Can you work these out from the model? Positions are in its coordinate system, mm. Face numbers are marked on the shaded views. A direction names the side the tool comes from. Round coordinates to 2 decimals unless told otherwise and drop trailing zeros. Order: outer loops, then holes, each group sorted by start corner. A loop starts at its lowest first (then second) coordinate and runs counter-clockwise, first axis right, second up. Notation, with made-up numbers: (77.25, -32.5) - (88.25, -32.5) arc R18 ccw to (88.25, -19.5) - close; hole circle Ø1 at (-9.5, -1.75). An arc over 180 degrees is marked (long way). Write item = value, one per line.
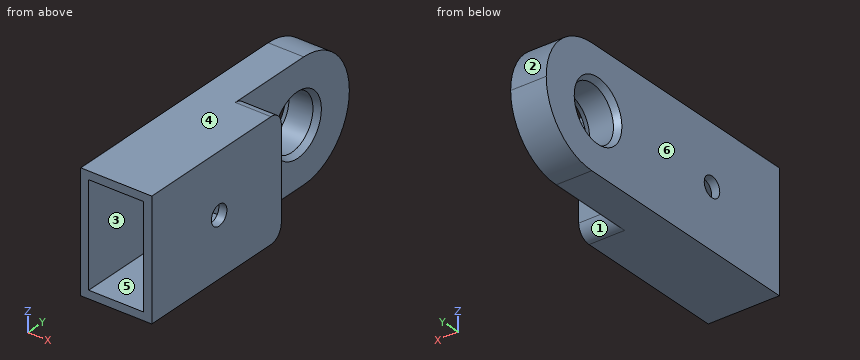
from build123d import *
from OCP.BRepFilletAPI import BRepFilletAPI_MakeChamfer

# Parameters (mm, degrees)
SKETCH1_W           = 10.6
SKETCH1_H           = 17.6
BOSS_EXTRUDE1_DEPTH = 25
SKETCH2_W           = 8.2
SKETCH2_H           = 15.2
CUT_EXTRUDE1_DEPTH  = 23
SKETCH4_W           = 5.3
SKETCH4_H           = 17.6
BOSS_EXTRUDE2_DEPTH = 20
CUT_EXTRUDE2_REACH  = 48.158
SKETCH5_R           = 4.1
FILLET1_R           = 8.8
FILLET2_R           = 2
SKETCH6_R           = 1.5
CUT_EXTRUDE3_DEPTH  = 48.061661679
CHAMFER1_SIZE       = 0.5
CHAMFER1_SIZE2      = 0.866025404


with BuildPart() as part:
    # Sketch1 → Boss-Extrude1 (new body)
    with BuildSketch(Plane(origin=(0, 0, 0), x_dir=(1, 0, 0), z_dir=(0, 1, 0))):
        Rectangle(SKETCH1_W, SKETCH1_H)
    extrude(amount=BOSS_EXTRUDE1_DEPTH)

    # Sketch2 → Cut-Extrude1 (cut)
    with BuildSketch(Plane.XZ):
        Rectangle(SKETCH2_W, SKETCH2_H)
    extrude(amount=-CUT_EXTRUDE1_DEPTH, mode=Mode.SUBTRACT)

    # Sketch4 → Boss-Extrude2 (add)
    with BuildSketch(Plane(origin=(0, 25, 0), x_dir=(1, 0, 0), z_dir=(0, 1, 0))):
        with Locations((-2.65, 0)):
            Rectangle(SKETCH4_W, SKETCH4_H)
    extrude(amount=BOSS_EXTRUDE2_DEPTH)

    # Sketch5 → Cut-Extrude2 (cut, up to next)
    with BuildSketch(Plane(origin=(0, 0, 0), x_dir=(0, 0, -1), z_dir=(1, 0, 0)), mode=Mode.PRIVATE) as cut_extrude2_sk1:
        with Locations((0, 35)):
            Circle(SKETCH5_R)
    cut_extrude2_tool1 = extrude(cut_extrude2_sk1.sketch, amount=-CUT_EXTRUDE2_REACH, mode=Mode.PRIVATE) & part.part
    add(cut_extrude2_tool1.solids().sort_by_distance((0, 35, 0))[0], mode=Mode.SUBTRACT)

    # Fillet1
    fillet1_edges = [part.edges().sort_by_distance(p)[0] for p in [
        (-2.65, 45, -8.8),
        (-2.65, 45, 8.8),
    ]]
    fillet(fillet1_edges, radius=FILLET1_R - 0.0001)  # a hair under: the kernel refuses the full size

    # Fillet2
    fillet2_edges = [part.edges().sort_by_distance(p)[0] for p in [
        (2.65, 25, 8.8),
        (2.65, 25, -8.8),
    ]]
    fillet(fillet2_edges, radius=FILLET2_R)

    # Sketch6 → Cut-Extrude3 (cut, through all)
    with BuildSketch(Plane(origin=(5.3, 0, 0), x_dir=(0, 0, -1), z_dir=(1, 0, 0))):
        with Locations((0, 13)):
            Circle(SKETCH6_R)
    extrude(amount=-CUT_EXTRUDE3_DEPTH, mode=Mode.SUBTRACT)

    # Chamfer1: one chamfer whose edges measure the first distance from different faces: ONE call of the kernel's chamfer builder (chamfer() names one face for all edges)
    chamfer1_edges_1 = [part.edges().sort_by_distance(p)[0] for p in [
        (0, 35, 4.1),
    ]]
    chamfer1_side_1 = [part.faces().sort_by_distance(p)[0] for p in [
        (0, 25.281737466, 0),
    ]]
    chamfer1_edges_2 = [part.edges().sort_by_distance(p)[0] for p in [
        (-5.3, 35, 4.1),
    ]]
    chamfer1_side_2 = [part.faces().sort_by_distance(p)[0] for p in [
        (-5.3, 20.674988238, 0),
    ]]
    chamfer1 = BRepFilletAPI_MakeChamfer(part.part.solid().wrapped)
    for e in chamfer1_edges_1:
        chamfer1.Add(CHAMFER1_SIZE, CHAMFER1_SIZE2, e.wrapped, chamfer1_side_1[0].wrapped)  # the first distance lies on this face
    for e in chamfer1_edges_2:
        chamfer1.Add(CHAMFER1_SIZE, CHAMFER1_SIZE2, e.wrapped, chamfer1_side_2[0].wrapped)  # the first distance lies on this face
    add(Compound.cast(chamfer1.Shape()), mode=Mode.REPLACE)


solid = part.part
(1) If we section it at A-A (y = 13): Write out the boundary of the cut face in (x, z), plus the area to 3 significant figures.
Computed:
outline = (-5.3, -8.8) - (5.3, -8.8) - (5.3, -1.5) - (4.1, -1.5) - (4.1, -7.6) - (-4.1, -7.6) - (-4.1, -1.5) - (-5.3, -1.5) - close; (-5.3, 1.5) - (-4.1, 1.5) - (-4.1, 7.6) - (4.1, 7.6) - (4.1, 1.5) - (5.3, 1.5) - (5.3, 8.8) - (-5.3, 8.8) - close
area = 54.7 mm^2
(2) Thinking about a two-plate mould opening in X: for the marked faces 3, 4, 5 and 6, which applies, +X half, -X half, draft (parallel to the pull), parting line (faces both ways), or undercut?
Computed:
face_3 = undercut
face_4 = draft
face_5 = undercut
face_6 = -X half
(3) If I drill on line 1 (X direction, y = 16, z = 3.75); line 2 (Z direction, x = -0.5, y = 13); line 3 (Y direction, x = 3, z = 4), over which ranges is the centre line in solid material (lowest first)? Write a range as from..to.
Computed:
line_1 = -5.3..-4.1, 4.1..5.3
line_2 = -8.8..-7.6, 7.6..8.8
line_3 = 23..25
(4) If we section it at D-D (z = 5.75): Write out the boundary of the cut face in (x, y), plus the area to 3 significant figures.
Computed:
outline = (-5.3, 0) - (-4.1, 0) - (-4.1, 23) - (4.1, 23) - (4.1, 0) - (5.3, 0) - (5.3, 25) - (0, 25) - (0, 42.86) - (-5.3, 42.86) - close
area = 171 mm^2
(5) Will these pins go through, and if not, where does the flat tip stop? P1, Ø5, axis at x = -1, z = -3, coming from the +Y side; P2, Ø5.5, axis at y = 37.5, z = 4, coming from the +X side; P3, Ø2.5, axis at y = 13, z = 0, coming from the -X side.
Computed:
P1 = 44.99
P2 = 0
P3 = through
(6) On a 3-axis mill with a long thin cutter (end or side, diameter ignored), from which of +Z, -Z, +X, -X, +Y, -Y can I reach the whole of each face in a straight line? I mean the marked faces 1 and 2. Say none if no direction works.
Computed:
face_1 = -Z, +X, +Y
face_2 = +Z, +X, -X, +Y
(7) If we section it at B-B (x = 3): Write out the boundary of the cut face in (y, z), plus the area to 3 significant figures.
Computed:
outline = (0, -8.8) - (23, -8.8) arc R2 ccw to (25, -6.8) - (25, 6.8) arc R2 ccw to (23, 8.8) - (0, 8.8) - (0, 7.6) - (23, 7.6) - (23, -7.6) - (0, -7.6) - close
area = 88.7 mm^2
(8) If we section it at C-C (y = 35): Write out the boundary of the cut face in (x, z).
Computed:
outline = (-5.3, -8.8) - (0, -8.8) - (0, -4.6) - (-0.87, -4.1) - (-4.43, -4.1) - (-5.3, -4.6) - close; (-5.3, 4.6) - (-4.43, 4.1) - (-0.87, 4.1) - (0, 4.6) - (0, 8.8) - (-5.3, 8.8) - close
